```python
from build123d import *
from build123d.topology import SkipClean

# Parameters (mm, degrees)
SKETCH1_R          = 3.4925
EXTRUDE1_DEPTH     = 0.5
EXTRUDE2_DEPTH     = 5.334
CUT_EXTRUDE1_REACH = 9.644
SKETCH3_R          = 0.88


with BuildPart() as part:
    # Sketch1 → Extrude1 (new body)
    with BuildSketch(Plane.XY):
        with Locations(Location((0, 0, 0), (0, 0, 133.702114437))):
            Circle(SKETCH1_R)
    extrude(amount=EXTRUDE1_DEPTH)

    # Sketch2 → Extrude2 (add)
    with SkipClean():  # the faces are left unmerged after this step: merging them gives an invalid solid
        with BuildSketch(Plane.XY.offset(0.5)):
            with BuildLine():
                Line((2.413, -2.52487371), (2.413, 2.52487371))
                ThreePointArc((2.413, 2.52487371), (0, 3.4925), (-2.413, 2.52487371))
                Line((-2.413, 2.52487371), (-2.413, -2.52487371))
                ThreePointArc((-2.413, -2.52487371), (0, -3.4925), (2.413, -2.52487371))
            make_face()
        extrude(amount=EXTRUDE2_DEPTH)

    # Sketch3 → Cut-Extrude1 (cut, up to next)
    with BuildSketch(Plane.XY.offset(5.834), mode=Mode.PRIVATE) as cut_extrude1_sk1:
        Circle(SKETCH3_R)
    cut_extrude1_tool1 = extrude(cut_extrude1_sk1.sketch, amount=-CUT_EXTRUDE1_REACH, mode=Mode.PRIVATE) & part.part
    add(cut_extrude1_tool1.solids().sort_by_distance((0, 0, 5.834))[0], mode=Mode.SUBTRACT)


solid = part.part
```
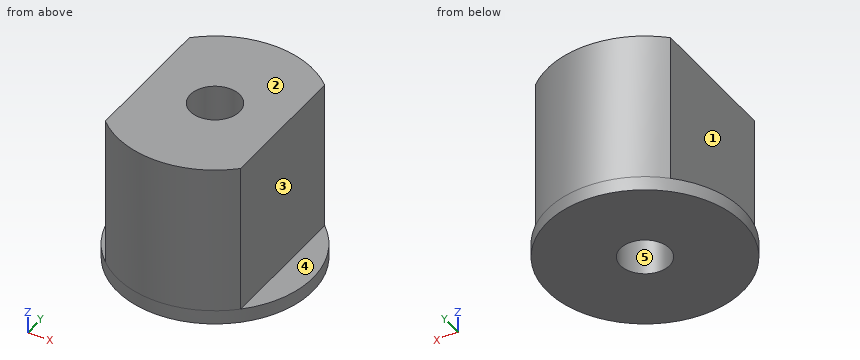
Could you check a few things on this model? Use its own coordinates, in mm. Face numbers are marked on the shaded views. A direction names the side the tool comes from. Coordinates: 2 decimals unless noted, no trailing zeros. Order: outer loops, then holes, each group sorted by start corner. A loop starts at its lowest first (then second) coordinate and runs counter-clockwise, first axis right, second up. Notation, with made-up numbers: M -40,-14.5 L -10,-14.5 A17 ccw -10,-9.5 Z; hole C 83,-12 d4. An arc over 180 degrees is marked long. Use a Markdown table: item, result. Add a question column.
Q1. I want a section at B-B on y = 0. List the corners of the cut face in (x, z) for me, then the cut area to 3 significant figures.
Q2. I want a section at D-D on y = -1.25. List the corners of the cut face in (x, z) for me, then the cut area to 3 significant figures.
Q3. I want a section at C-C on x = 0. List the corners of the cut face in (y, z) for me.
Q4. Which directions (+Z, -Z, +X, -X, +Y, -Y) give clear straight access to the entire face, cutting with the end or side of a thin tool? Please do the marked faces 1, 2 and 3.
Q5. If I drill on L1, parallel to Y at x = 0, z = 1.9; L2, parallel to X at y = -2.25, z = 4.8; L3, parallel to Y at x = -0.5, z = 2.35, over which ranges is the centre line in solid material (lowest first)?
Q6. I'm going to push flat-ended pins straight in: pin 1 (2 mm diameter, centred on y = -1.5, z = 5, fed in from -X); pin 2 (1.1 mm diameter, centred on x = 0, y = 0, fed in from -Z); pin 3 (0.5 mm diameter, centred on x = -3, y = -0.5, fed in from +Z). Where does each tip first touch, or does it pass through?
Q7. I want a section at A-A on z = 1.3. List the corners of the cut face in (x, y) for me (1 decimal), then the cut area to 3 significant figures.
Q8. We'd pull the mould along Y, two halves only. Please class the marked faces 4 and 5: pulls with the +Y half, pulls with the -Y half, needs draft (parallel to the pull), parting line crosses it, or undercut.
Checked values:
| question | item | result |
|---|---|---|
| 1 | outline | M -3.49,0 L -0.88,0 L -0.88,5.83 L -2.41,5.83 L -2.41,0.5 L -3.49,0.5 Z; M 0.88,0 L 3.49,0 L 3.49,0.5 L 2.41,0.5 L 2.41,5.83 L 0.88,5.83 Z |
| 1 | area | 19.0 mm² |
| 2 | outline | M -3.26,0 L 3.26,0 L 3.26,0.5 L 2.41,0.5 L 2.41,5.83 L -2.41,5.83 L -2.41,0.5 L -3.26,0.5 Z |
| 2 | area | 29.0 mm² |
| 3 | outline | M -3.49,0 L -0.88,0 L -0.88,5.83 L -3.49,5.83 Z; M 0.88,0 L 3.49,0 L 3.49,5.83 L 0.88,5.83 Z |
| 4 | face 1 | +Z, -X, +Y, -Y |
| 4 | face 2 | +Z, +X, -X, +Y, -Y |
| 4 | face 3 | +Z, +X, +Y, -Y |
| 5 | L1 | -3.49 to -0.88, 0.88 to 3.49 |
| 5 | L2 | -2.41 to 2.41 |
| 5 | L3 | -3.46 to -0.72, 0.72 to 3.46 |
| 6 | pin 1 | x = -2.41 |
| 6 | pin 2 | through |
| 6 | pin 3 | z = 0.5 |
| 7 | outline | M -2.4,-2.5 A3.5 ccw 2.4,-2.5 L 2.4,2.5 A3.5 ccw -2.4,2.5 Z; hole C 0,0 d1.8 |
| 7 | area | 28.4 mm² |
| 8 | face 4 | needs draft |
| 8 | face 5 | undercut |
